Can you work these out from the model? Positions are in its coordinate system, mm. Face numbers are marked on the shaded views. A direction names the side the tool comes from. Give positions to 0.01 mm unless a question says otherwise; leave off trailing zeros. Write each loop counter-clockwise with the first axis right and the second up, starting at its lowest first coordinate (ties: lowest second). Pieces come first, ordered by that corner, then holes. Notation, with made-up numbers: (30, 48) - (39, 48) arc R25 ccw to (39, 77) - close; hole circle Ø11 at (24.5, 48). An arc over 180 degrees is marked (long way). Return JSON: item names as keys, results as strings. Group by question number.
from build123d import *

# Parameters (mm, degrees)
SKETCH1_R           = 75
BOSS_EXTRUDE1_DEPTH = 125
FILLET1_R           = 50
SKETCH2_R           = 12.5
CUT_EXTRUDE1_DEPTH  = 441.624556737


with BuildPart() as part:
    # Sketch1 → Boss-Extrude1 (new, symmetric)
    with BuildSketch(Plane.XY):
        with BuildLine():
            Line((-106, 0), (-106, 132))
            Line((-106, 132), (-325, 132))
            Line((-325, 132), (-325, 164))
            Line((-325, 164), (325, 164))
            Line((325, 164), (325, 132))
            Line((325, 132), (106, 132))
            Line((106, 132), (106, 0))
            ThreePointArc((106, 0), (0, -106), (-106, 0))
        make_face()
        Circle(SKETCH1_R, mode=Mode.SUBTRACT)
    extrude(amount=BOSS_EXTRUDE1_DEPTH, both=True)

    # Fillet1
    fillet1_edges = [part.edges().sort_by_distance(p)[0] for p in [
        (106, 132, 0),
        (-106, 132, 0),
    ]]
    fillet(fillet1_edges, radius=FILLET1_R)

    # Sketch2 → Cut-Extrude1 (cut, through all)
    with BuildSketch(Plane(origin=(0, 164, 0), x_dir=(1, 0, 0), z_dir=(0, 1, 0))):
        with Locations(Location((-250, 62.5, 0), (0, 0, 180))):
            Circle(SKETCH2_R)
        with Locations(Location((-250, -62.5, 0), (0, 0, 180))):
            Circle(SKETCH2_R)
        with Locations(Location((250, -62.5, 0), (0, 0, 180))):
            Circle(SKETCH2_R)
        with Locations(Location((250, 62.5, 0), (0, 0, 180))):
            Circle(SKETCH2_R)
    extrude(amount=-CUT_EXTRUDE1_DEPTH, mode=Mode.SUBTRACT)


solid = part.part
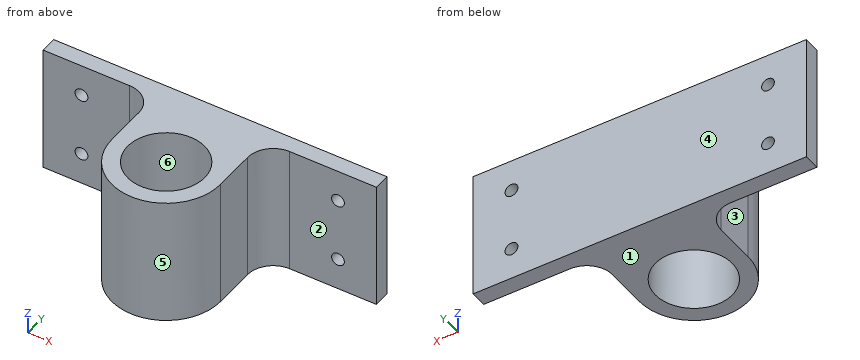
1) Imagine slicing it at A-A, the plane z = 62.5. Write out the boundary of the cut face in (x, y).
2) On a 3-axis mill with a long thin cutter (end or side, diameter ignored), from which of +Z, -Z, +X, -X, +Y, -Y can I reach the whole of each face in a straight line? I mean the marked faces 1, 2 and 3. Say none if no direction works.
3) I need wall thicknesses on line 1 along X through (y, z) = (153, -62); line 2 along Z through (x, y) = (250, 148); line 3 along Y through (x, z) = (0, -23). Which ranges of each line are inside material? Lowest first, please.
4) Imagine slicing it at C-C, the plane z = -81. Write out the boundary of the cut face in (x, y), and give its area (3 significant figures).
5) Imagine slicing it at B-B, the plane x = 0. Write out the boundary of the cut face in (y, z).
6) Imagine slicing it at D-D, the plane x = 249.5. Write out the boundary of the cut face in (y, z).
7) Will these pins go through, and if not, where does the flat tip stop? pin 1 Ø12 at (x, z) = (178, 99.5) entering from -Y; pin 2 Ø12 at (y, z) = (94.5, -41) entering from -X; pin 3 Ø1.5 at (y, z) = (83, -11) entering from +X.
8) We'd pull the mould along Y, two halves only. Please class the marked faces 4, 5 and 6: pulls with the +Y half, pulls with the -Y half, needs draft (parallel to the pull), parting line crosses it, or undercut.
Resolved:
{
 "1": {"outline": "(-325, 132) - (-262.5, 132) - (-262.5, 164) - (-325, 164) - close; (-237.5, 132) - (-156, 132) arc R50 cw to (-106, 82) - (-106, 0) arc R106 ccw to (106, 0) - (106, 82) arc R50 cw to (156, 132) - (237.5, 132) - (237.5, 164) - (-237.5, 164) - close; (262.5, 132) - (325, 132) - (325, 164) - (262.5, 164) - close; hole circle Ø150 at (0, 0)"},
 "2": {"face 1": "-Z, +X, -X, +Y, -Y", "face 2": "+Z, -Z, +X, -Y", "face 3": "+Z, -Z, -X, -Y"},
 "3": {"line 1": "-325 to -262.49, -237.51 to 237.51, 262.49 to 325", "line 2": "-125 to -75, -50 to 50, 75 to 125", "line 3": "-106 to -75, 75 to 164"},
 "4": {"outline": "(-325, 132) - (-156, 132) arc R50 cw to (-106, 82) - (-106, 0) arc R106 ccw to (106, 0) - (106, 82) arc R50 cw to (156, 132) - (325, 132) - (325, 164) - (-325, 164) - close; hole circle Ø150 at (0, 0)", "area": "49,800 mm^2"},
 "5": {"outline": "(-106, -125) - (-75, -125) - (-75, 125) - (-106, 125) - close; (75, -125) - (164, -125) - (164, 125) - (75, 125) - close"},
 "6": {"outline": "(132, -125) - (164, -125) - (164, -74.99) - (132, -74.99) - close; (132, -50.01) - (164, -50.01) - (164, 50.01) - (132, 50.01) - close; (132, 74.99) - (164, 74.99) - (164, 125) - (132, 125) - close"},
 "7": {"pin 1": "y = 132", "pin 2": "x = -109.55", "pin 3": "x = 106.03"},
 "8": {"face 4": "pulls with the +Y half", "face 5": "pulls with the -Y half", "face 6": "undercut"}
}
